```python
from build123d import *


with BuildPart() as part:
    # Sketch1 → Revolve1 (revolve)
    with BuildSketch(Plane.XY):
        with BuildLine():
            Line((4.7625, 0), (4.7625, 15.937))
            ThreePointArc((4.7625, 15.937), (4.911289755, 16.296210245), (5.2705, 16.445))
            Line((5.2705, 16.445), (9.434996824, 16.445))
            ThreePointArc((9.434996824, 16.445), (9.75286634, 16.333261241), (9.930899851, 16.047200673))
            Line((9.930899851, 16.047200673), (12.370403027, 5.06943638))
            ThreePointArc((12.370403027, 5.06943638), (12.379466701, 5.014667028), (12.3825, 4.959235708))
            Line((12.3825, 4.959235708), (12.3825, 0))
            Line((12.3825, 0), (4.7625, 0))
        make_face()
    revolve(axis=Axis((0, 0, 0), (0, 1, 0)))


solid = part.part
```
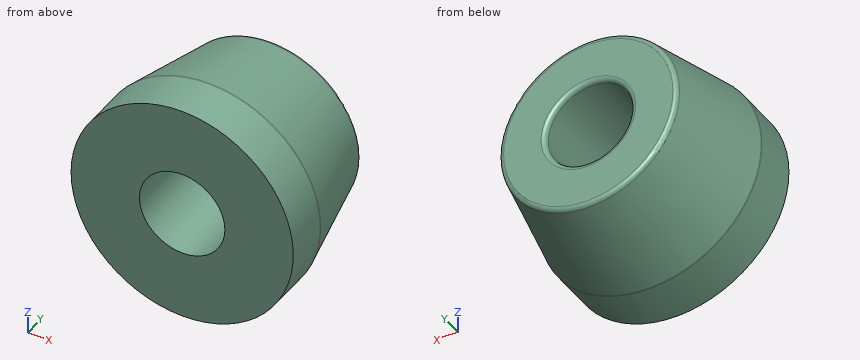
Could you check a few things on this model? Use its own coordinates, in mm. Round coordinates to 2 decimals unless told otherwise and drop trailing zeros. Loops run counter-clockwise (first coordinate to the right, second up) from the corner with the lowest first, then second, coordinate; pieces in that order, holes last. Notation, with made-up numbers: (-9, 38) - (33, 38) arc R23 cw to (33, 70) - close; hole circle Ø11 at (-15.5, 79). An arc over 180 degrees is marked (long way). Answer in a Markdown table with one row per item. Add a question column.
(1) I need wall thicknesses on line 1 along Z through (x, y) = (0, 5); line 2 along X through (y, z) = (8, -1.75); line 3 along X through (y, z) = (9.25, -2.5). Which ranges of each line are inside material? Lowest first, please.
(2) I'm going to push flat-ended pins straight in: pin 1 (2 mm diameter, centred on y = 6.5, z = 1, fed in from -X); pin 2 (8 mm diameter, centred on y = 4, z = -9.5, fed in from -X); pin 3 (6 mm diameter, centred on y = 12.5, z = -0.5, fed in from +X). Where does each tip first touch, or does it pass through?
(3) If we section it at D-D (y = 13.25): Please give me the cut outline in (x, z) (1 decimal), plus the area to 3 significant figures.
(4) If we section it at C-C (y = 1): Please give me the cut outline in (x, z) (1 decimal).
Model answer:
| question | item | result |
|---|---|---|
| 1 | line 1 | z = -12.38 to -4.76, 4.76 to 12.38 |
| 1 | line 2 | x = -11.59 to -4.43, 4.43 to 11.59 |
| 1 | line 3 | x = -11.16 to -4.05, 4.05 to 11.16 |
| 2 | pin 1 | stops at x = -12.24 |
| 2 | pin 2 | stops at x = -11.09 |
| 2 | pin 3 | stops at x = 11.38 |
| 3 | outline | circle Ø21.1 at (0, 0); hole circle Ø9.5 at (0, 0) |
| 3 | area | 279 mm² |
| 4 | outline | circle Ø24.8 at (0, 0); hole circle Ø9.5 at (0, 0) |
